Here's how the part is built. I have some questions about the finished solid (model axes, mm). Coordinates: 2 decimals unless noted, no trailing zeros. Write each loop counter-clockwise with the first axis right and the second up, starting at its lowest first coordinate (ties: lowest second). Pieces come first, ordered by that corner, then holes. Notation, with made-up numbers: (53, 15) -> (94, 15) arc R35 cw to (94, 53) -> close; hole circle Ø1 at (89.25, 81). An arc over 180 degrees is marked (long way). Put each result on its own line as item: value. Start each with the question number.
Item 1: I want a section at B-B, the plane x = 8.5. List the corners of the cut face in (y, z) for me, then the cut area to 3 significant figures.
Item 2: I need wall thicknesses on line 1 (Z direction, x = 17, y = 1.85); line 2 (X direction, y = 1.7, z = 6.5); line 3 (Z direction, x = 10, y = 1.95). Which ranges of each line are inside material? Lowest first, please. Write a range as [from, to].
Item 3: For pin 1 (6 mm diameter, centred on x = -11.5, z = 0.5, fed in from -Y); pin 2 (1 mm diameter, centred on x = 16.5, z = -2, fed in from +Y), each with a flat end and sliding along its axis, tell me the tip position at first contact or that it passes through.
Item 4: I want a section at C-C, the plane y = 0.9. List the corners of the cut face in (x, z) for me.
Item 5: I want a section at A-A, the plane z = 0. List the corners of the cut face in (x, y) for me.
from build123d import *

# Parameters (mm, degrees)
SKETCH1_W           = 50.8
SKETCH1_H           = 50.8
BOSS_EXTRUDE1_DEPTH = 2.54
CUT_EXTRUDE2_DEPTH  = 2.54


with BuildPart() as part:
    # Sketch1 → Boss-Extrude1 (new body)
    with BuildSketch(Plane(origin=(0, 0, 0), x_dir=(1, 0, 0), z_dir=(0, 1, 0))):
        Rectangle(SKETCH1_W, SKETCH1_H)
    extrude(amount=BOSS_EXTRUDE1_DEPTH)

    # Sketch2 → Cut-Extrude2 (cut)
    with BuildSketch(Plane.XZ):
        with BuildLine():
            Line((-4.214616619, 6.877540553), (-6.799823365, 4.227137698))
            Line((-6.799823365, 4.227137698), (-17.756833433, 2.46184495))
            ThreePointArc((-17.756833433, 2.46184495), (-19.612357967, 0), (-17.756833433, -2.46184495))
            Line((-17.756833433, -2.46184495), (-6.799823365, -4.227137698))
            Line((-6.799823365, -4.227137698), (-4.214616619, -6.877540553))
            Line((-4.214616619, -6.877540553), (-2.46184495, -17.756833433))
            ThreePointArc((-2.46184495, -17.756833433), (0, -19.612357967), (2.46184495, -17.756833433))
            Line((2.46184495, -17.756833433), (4.214616619, -6.877540553))
            Line((4.214616619, -6.877540553), (6.799823365, -4.227137698))
            Line((6.799823365, -4.227137698), (17.756833433, -2.46184495))
            ThreePointArc((17.756833433, -2.46184495), (19.612357967, 0), (17.756833433, 2.46184495))
            Line((17.756833433, 2.46184495), (6.877540553, 4.214616619))
            Line((6.877540553, 4.214616619), (4.227137698, 6.799823365))
            Line((4.227137698, 6.799823365), (2.558814736, 17.15495087))
            ThreePointArc((2.558814736, 17.15495087), (2.557405809, 17.185318827), (2.555636489, 17.21566792))
            ThreePointArc((2.555636489, 17.21566792), (0.274616535, 19.597591266), (-2.46184495, 17.756833433))
            Line((-2.46184495, 17.756833433), (-4.214616619, 6.877540553))
        make_face()
    extrude(amount=-CUT_EXTRUDE2_DEPTH, mode=Mode.SUBTRACT)


solid = part.part
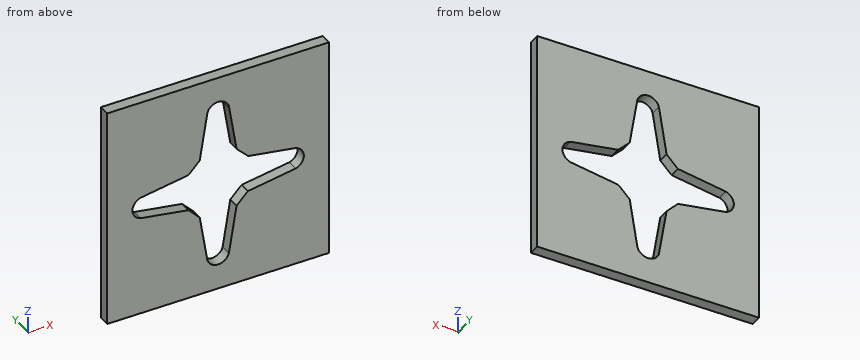
Calculated:
1. outline: (0, -25.4) -> (2.54, -25.4) -> (2.54, -3.95) -> (0, -3.95) -> close; (0, 3.95) -> (2.54, 3.95) -> (2.54, 25.4) -> (0, 25.4) -> close
1. area: 109 mm2
2. line 1: z = [-25.4, -2.58], [2.58, 25.4]
2. line 2: x = [-25.4, -4.58], [4.53, 25.4]
2. line 3: z = [-25.4, -3.71], [3.71, 25.4]
3. pin 1: stops at y = 0
3. pin 2: passes through
4. outline: (-25.4, -25.4) -> (25.4, -25.4) -> (25.4, 25.4) -> (-25.4, 25.4) -> close; hole (-17.76, -2.46) -> (-6.8, -4.23) -> (-4.21, -6.88) -> (-2.46, -17.76) arc R2.56 ccw to (2.46, -17.76) -> (4.21, -6.88) -> (6.8, -4.23) -> (17.76, -2.46) arc R2.56 ccw to (17.76, 2.46) -> (6.88, 4.21) -> (4.23, 6.8) -> (2.56, 17.15) arc R2.56 ccw to (2.56, 17.22) arc R2.56 ccw to (-2.46, 17.76) -> (-4.21, 6.88) -> (-6.8, 4.23) -> (-17.76, 2.46) arc R2.56 ccw to start
5. outline: (-25.4, 0) -> (-19.61, 0) -> (-19.61, 2.54) -> (-25.4, 2.54) -> close; (19.61, 0) -> (25.4, 0) -> (25.4, 2.54) -> (19.61, 2.54) -> close
